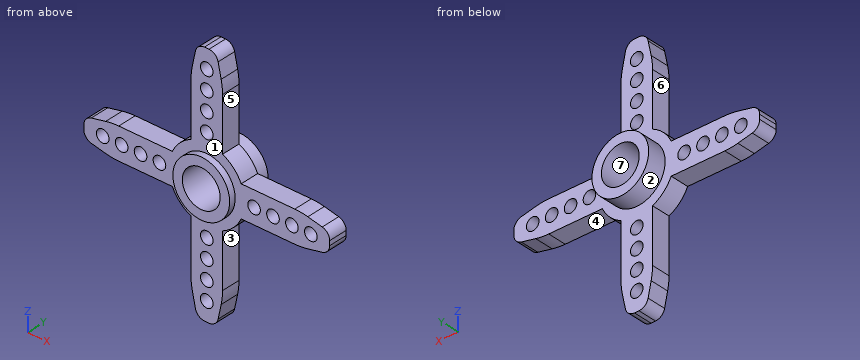
from build123d import *

# Parameters (mm, degrees)
SKETCH1_R           = 4.5
SKETCH1_R_2         = 1
BOSS_EXTRUDE1_DEPTH = 3
SKETCH1_4_R         = 4.5
SKETCH1_4_R_2       = 3
BOSS_EXTRUDE2_DEPTH = 6
BOSS_EXTRUDE3_START = -1
SKETCH1_5_R         = 4.5
SKETCH1_5_R_2       = 3
BOSS_EXTRUDE3_DEPTH = 1


with BuildPart() as part:
    # Sketch1 → Boss-Extrude1 (new body)
    with BuildSketch(Plane(origin=(0, 0, 0), x_dir=(1, 0, 0), z_dir=(0, 1, 0))):
        with BuildLine():
            Line((-1.800704436, 18.307444008), (-2.283369641, 16.026447288))
            ThreePointArc((-2.283369641, 16.026447288), (-2.445694958, 14.997005048), (-2.5, 13.956259259))
            Line((-2.5, 13.956259259), (-2.5, 5.454356057))
            ThreePointArc((-2.5, 5.454356057), (-4.242640687, 4.242640687), (-5.454356057, 2.5))
            Line((-5.454356057, 2.5), (-13.956259259, 2.5))
            ThreePointArc((-13.956259259, 2.5), (-14.997005048, 2.445694958), (-16.026447288, 2.283369641))
            Line((-16.026447288, 2.283369641), (-18.307444008, 1.800704436))
            ThreePointArc((-18.307444008, 1.800704436), (-19.153411563, 1.288456839), (-19.496658787, 0.360965573))
            ThreePointArc((-19.496658787, 0.360965573), (-19.5, 0), (-19.496658787, -0.360965573))
            ThreePointArc((-19.496658787, -0.360965573), (-19.153411563, -1.288456839), (-18.307444008, -1.800704436))
            Line((-18.307444008, -1.800704436), (-16.026447288, -2.283369641))
            ThreePointArc((-16.026447288, -2.283369641), (-14.997005048, -2.445694958), (-13.956259259, -2.5))
            Line((-13.956259259, -2.5), (-5.454356057, -2.5))
            ThreePointArc((-5.454356057, -2.5), (-4.242640687, -4.242640687), (-2.5, -5.454356057))
            Line((-2.5, -5.454356057), (-2.5, -13.956259259))
            ThreePointArc((-2.5, -13.956259259), (-2.445694958, -14.997005048), (-2.283369641, -16.026447288))
            Line((-2.283369641, -16.026447288), (-1.800704436, -18.307444008))
            ThreePointArc((-1.800704436, -18.307444008), (-1.288456839, -19.153411563), (-0.360965573, -19.496658787))
            ThreePointArc((-0.360965573, -19.496658787), (0, -19.5), (0.360965573, -19.496658787))
            ThreePointArc((0.360965573, -19.496658787), (1.288456839, -19.153411563), (1.800704436, -18.307444008))
            Line((1.800704436, -18.307444008), (2.283369641, -16.026447288))
            ThreePointArc((2.283369641, -16.026447288), (2.445694958, -14.997005048), (2.5, -13.956259259))
            Line((2.5, -13.956259259), (2.5, -5.454356057))
            ThreePointArc((2.5, -5.454356057), (4.242640687, -4.242640687), (5.454356057, -2.5))
            Line((5.454356057, -2.5), (13.956259259, -2.5))
            ThreePointArc((13.956259259, -2.5), (14.997005048, -2.445694958), (16.026447288, -2.283369641))
            Line((16.026447288, -2.283369641), (18.307444008, -1.800704436))
            ThreePointArc((18.307444008, -1.800704436), (19.153411563, -1.288456839), (19.496658787, -0.360965573))
            ThreePointArc((19.496658787, -0.360965573), (19.5, 0), (19.496658787, 0.360965573))
            ThreePointArc((19.496658787, 0.360965573), (19.153411563, 1.288456839), (18.307444008, 1.800704436))
            Line((18.307444008, 1.800704436), (16.026447288, 2.283369641))
            ThreePointArc((16.026447288, 2.283369641), (14.997005048, 2.445694958), (13.956259259, 2.5))
            Line((13.956259259, 2.5), (5.454356057, 2.5))
            ThreePointArc((5.454356057, 2.5), (4.242640687, 4.242640687), (2.5, 5.454356057))
            Line((2.5, 5.454356057), (2.5, 13.956259259))
            ThreePointArc((2.5, 13.956259259), (2.445694958, 14.997005048), (2.283369641, 16.026447288))
            Line((2.283369641, 16.026447288), (1.800704436, 18.307444008))
            ThreePointArc((1.800704436, 18.307444008), (1.288456839, 19.153411563), (0.360965573, 19.496658787))
            ThreePointArc((0.360965573, 19.496658787), (0, 19.5), (-0.360965573, 19.496658787))
            ThreePointArc((-0.360965573, 19.496658787), (-1.288456839, 19.153411563), (-1.800704436, 18.307444008))
        make_face()
        with Locations(Location((0, 0, 0), (0, 0, 270))):
            Circle(SKETCH1_R, mode=Mode.SUBTRACT)
        with Locations(Location((0, 7.5, 0), (0, 0, 270))):
            Circle(SKETCH1_R_2, mode=Mode.SUBTRACT)
        with Locations(Location((0, 10.5, 0), (0, 0, 270))):
            Circle(SKETCH1_R_2, mode=Mode.SUBTRACT)
        with Locations(Location((0, 13.5, 0), (0, 0, 270))):
            Circle(SKETCH1_R_2, mode=Mode.SUBTRACT)
        with Locations(Location((0, 16.5, 0), (0, 0, 270))):
            Circle(SKETCH1_R_2, mode=Mode.SUBTRACT)
        with Locations(Location((7.5, 0, 0), (0, 0, 270))):
            Circle(SKETCH1_R_2, mode=Mode.SUBTRACT)
        with Locations(Location((10.5, 0, 0), (0, 0, 270))):
            Circle(SKETCH1_R_2, mode=Mode.SUBTRACT)
        with Locations(Location((13.5, 0, 0), (0, 0, 270))):
            Circle(SKETCH1_R_2, mode=Mode.SUBTRACT)
        with Locations(Location((16.5, 0, 0), (0, 0, 270))):
            Circle(SKETCH1_R_2, mode=Mode.SUBTRACT)
        with Locations(Location((0, -7.5, 0), (0, 0, 270))):
            Circle(SKETCH1_R_2, mode=Mode.SUBTRACT)
        with Locations(Location((0, -10.5, 0), (0, 0, 270))):
            Circle(SKETCH1_R_2, mode=Mode.SUBTRACT)
        with Locations(Location((0, -13.5, 0), (0, 0, 270))):
            Circle(SKETCH1_R_2, mode=Mode.SUBTRACT)
        with Locations(Location((0, -16.5, 0), (0, 0, 270))):
            Circle(SKETCH1_R_2, mode=Mode.SUBTRACT)
        with Locations(Location((-7.5, 0, 0), (0, 0, 270))):
            Circle(SKETCH1_R_2, mode=Mode.SUBTRACT)
        with Locations(Location((-10.5, 0, 0), (0, 0, 270))):
            Circle(SKETCH1_R_2, mode=Mode.SUBTRACT)
        with Locations(Location((-13.5, 0, 0), (0, 0, 270))):
            Circle(SKETCH1_R_2, mode=Mode.SUBTRACT)
        with Locations(Location((-16.5, 0, 0), (0, 0, 270))):
            Circle(SKETCH1_R_2, mode=Mode.SUBTRACT)
    extrude(amount=BOSS_EXTRUDE1_DEPTH)

    # Sketch1_4 → Boss-Extrude2 (add)
    with BuildSketch(Plane(origin=(0, 0, 0), x_dir=(1, 0, 0), z_dir=(0, 1, 0))):
        with Locations(Location((0, 0, 0), (0, 0, 270))):
            Circle(SKETCH1_4_R)
        with Locations(Location((0, 0, 0), (0, 0, 270))):
            Circle(SKETCH1_4_R_2, mode=Mode.SUBTRACT)
    extrude(amount=BOSS_EXTRUDE2_DEPTH)

    # Sketch1_5 → Boss-Extrude3 (add)
    with BuildSketch(Plane(origin=(0, 0, 0), x_dir=(1, 0, 0), z_dir=(0, 1, 0)).offset(BOSS_EXTRUDE3_START)):
        with Locations(Location((0, 0, 0), (0, 0, 270))):
            Circle(SKETCH1_5_R)
        with Locations(Location((0, 0, 0), (0, 0, 270))):
            Circle(SKETCH1_5_R_2, mode=Mode.SUBTRACT)
    extrude(amount=BOSS_EXTRUDE3_DEPTH)


solid = part.part
For this review, take the finished solid that the model builds, in its own axes (mm). Face numbers are marked on the shaded views. A direction names the side the tool comes from. Round coordinates to 2 decimals unless told otherwise and drop trailing zeros. Write each loop counter-clockwise with the first axis right and the second up, starting at its lowest first coordinate (ties: lowest second). Pieces come first, ordered by that corner, then holes. Notation, with made-up numbers: M -25.75,80.5 L -3.75,80.5 A29 ccw -3.75,107.5 Z; hole C 85,58.5 d4. An arc over 180 degrees is marked long. Write item = value, one per line. Start each with the question number.
(1) For the marked faces 1, 2 and 3, list the 3-axis set-ups (+Z, -Z, +X, -X, +Y, -Y) from which the entire face can be reached by the end or side of a thin tool; tool diameter is ignored.
(2) The part is to be moulded in two halves that separate along X. For the marked faces 4, 5, 6 and 7, say which applies: +X half, -X half, draft (parallel to the pull), parting line (faces both ways), or undercut.
(3) Clearance check with flat-ended pins moving along their axes: pin 1 Ø1.8 at (x, z) = (16.5, 0) entering from -Y; pin 2 Ø0.9 at (y, z) = (2, -8.5) entering from +X; pin 3 Ø1 at (x, y) = (-12, 0.5) entering from +Z; pin 4 Ø2.5 at (x, z) = (10.5, 0) entering from +Y. State where each tip first meets the part, or that it passes through.
(4) We need section C-C (y = 3.5). Give the boundary of the cut face in (x, z).
(5) We need section D-D (x = 15). Give the boundary of the cut face in (y, z), then the cut area to 3 significant figures.
(6) For line 1 along X through (y, z) = (1.4, 10.5); line 2 along X through (y, z) = (4.25, 0); line 3 along Z through (x, y) = (12, 0.75), list the stretches that pass through material, from the lowest coordinate up.
(7) We need section B-B (z = 7.5). Give the boundary of the cut face in (x, y).
(8) We need section A-A (x = 7.5). Give the boundary of the cut face in (y, z).
Results found:
q1.face_1 = -Y
q1.face_2 = +Y
q1.face_3 = -Z, +X, +Y, -Y
q2.face_4 = draft
q2.face_5 = +X half
q2.face_6 = -X half
q2.face_7 = undercut
q3.pin_1 = through
q3.pin_2 = 2.5
q3.pin_3 = 2.5
q3.pin_4 = 3
q4.outline = C 0,0 d9; hole C 0,0 d6
q5.outline = M 0,-2.45 L 3,-2.45 L 3,2.45 L 0,2.45 Z
q5.area = 14.7 mm²
q6.line_1 = -2.5 to -1, 1 to 2.5
q6.line_2 = -4.5 to -3, 3 to 4.5
q6.line_3 = -2.5 to 2.5
q7.outline = M -2.5,0 L -1,0 L -1,3 L -2.5,3 Z; M 1,0 L 2.5,0 L 2.5,3 L 1,3 Z
q8.outline = M 0,-2.5 L 3,-2.5 L 3,-1 L 0,-1 Z; M 0,1 L 3,1 L 3,2.5 L 0,2.5 Z
